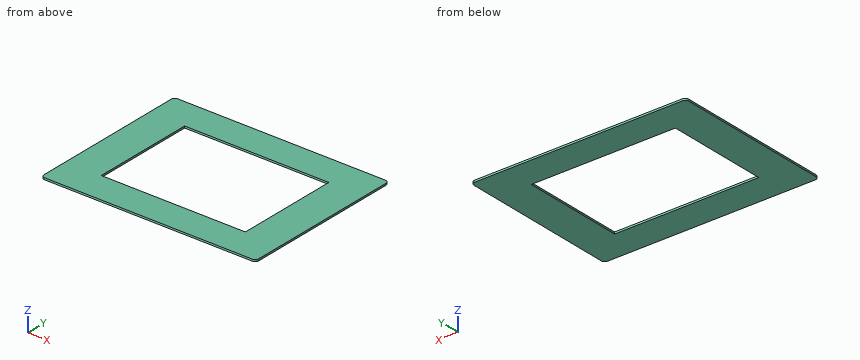
from build123d import *

# Parameters (mm, degrees)
SKETCH1_W           = 295
SKETCH1_H           = 225
SKETCH1_W_2         = 198
SKETCH1_H_2         = 141
BOSS_EXTRUDE1_DEPTH = 2.5
FILLET1_R           = 5


with BuildPart() as part:
    # Sketch1 → Boss-Extrude1 (new body)
    with BuildSketch(Plane.XY):
        Rectangle(SKETCH1_W, SKETCH1_H)
        Rectangle(SKETCH1_W_2, SKETCH1_H_2, mode=Mode.SUBTRACT)
    extrude(amount=BOSS_EXTRUDE1_DEPTH)

    # Fillet1
    fillet1_edges = [part.edges().sort_by_distance(p)[0] for p in [
        (147.5, -112.5, 1.25),
        (-147.5, -112.5, 1.25),
        (-147.5, 112.5, 1.25),
        (147.5, 112.5, 1.25),
    ]]
    fillet(fillet1_edges, radius=FILLET1_R)


solid = part.part
Geometry: final body of the model. Coordinates: model frame, mm. Coordinates: 2 decimals unless noted, no trailing zeros. Order: outer loops, then holes, each group sorted by start corner. A loop starts at its lowest first (then second) coordinate and runs counter-clockwise, first axis right, second up.
(1) Section query C-C (x = 78.5). Return the cut outline in (y, z), plus the area to 3 significant figures.
(2) Material intervals for probe 1 along Y at (x, z) = (81.5, 2.05); probe 2 along X at (y, z) = (-69.5, 1.8), sorted ascending.
(3) Section query B-B (y = 15). Return the cut outline in (x, z), plus the area to 4 significant figures.
(4) Section query A-A (z = 0.8). Return the cut outline in (x, y).
Solution:
1. outline: (-112.5, 0) - (-70.5, 0) - (-70.5, 2.5) - (-112.5, 2.5) - close; (70.5, 0) - (112.5, 0) - (112.5, 2.5) - (70.5, 2.5) - close
1. area: 210 mm2
2. probe 1: y = -112.5 to -70.5, 70.5 to 112.5
2. probe 2: x = -147.5 to -99, 99 to 147.5
3. outline: (-147.5, 0) - (-99, 0) - (-99, 2.5) - (-147.5, 2.5) - close; (99, 0) - (147.5, 0) - (147.5, 2.5) - (99, 2.5) - close
3. area: 242.5 mm2
4. outline: (-147.5, -107.5) arc R5 ccw to (-142.5, -112.5) - (142.5, -112.5) arc R5 ccw to (147.5, -107.5) - (147.5, 107.5) arc R5 ccw to (142.5, 112.5) - (-142.5, 112.5) arc R5 ccw to (-147.5, 107.5) - close; hole (-99, -70.5) - (99, -70.5) - (99, 70.5) - (-99, 70.5) - close
